```python
from build123d import *

# Parameters (mm, degrees)
SKETCH1_R           = 2
BOSS_EXTRUDE1_DEPTH = 8
SKETCH2_R           = 7.5
SKETCH2_R_2         = 4.5
BOSS_EXTRUDE2_DEPTH = 8
SKETCH3_R           = 2
BOSS_EXTRUDE3_DEPTH = 8
SKETCH8_W           = 30
SKETCH8_H           = 8
BOSS_EXTRUDE7_DEPTH = 15.35
BOSS_EXTRUDE8_DEPTH = 30
BOSS_EXTRUDE9_DEPTH = 8


with BuildPart() as part:
    # Sketch1 → Boss-Extrude1 (new body)
    with BuildSketch(Plane.XY):
        with BuildLine():
            Line((134.5, -11.9), (174.5, -11.9))
            ThreePointArc((174.5, -11.9), (182, -19.4), (174.5, -26.9))
            Line((174.5, -26.9), (134.5, -26.9))
            ThreePointArc((134.5, -26.9), (127, -19.4), (134.5, -11.9))
        make_face()
        with Locations((134.5, -19.4)):
            Circle(SKETCH1_R, mode=Mode.SUBTRACT)
        with Locations((174.5, -19.4)):
            Circle(SKETCH1_R, mode=Mode.SUBTRACT)
    extrude(amount=BOSS_EXTRUDE1_DEPTH)

    # Sketch8 → Boss-Extrude7 (add)
    with BuildSketch(Plane(origin=(0, -26.9, 0), x_dir=(-1, 0, 0), z_dir=(0, -1, 0))):
        with Locations((-154.2, -4)):
            Rectangle(SKETCH8_W, SKETCH8_H)
    extrude(amount=BOSS_EXTRUDE7_DEPTH)



with BuildPart() as body_2:
    # Sketch2 → Boss-Extrude2 (new body)
    with BuildSketch(Plane(origin=(0, -42.25, 0), x_dir=(1, 0, 0), z_dir=(0, 1, 0))):
        with Locations(Location((154.2, -16, 0), (0, 0, 270))):
            Circle(SKETCH2_R)
        with Locations(Location((154.2, -16, 0), (0, 0, 270))):
            Circle(SKETCH2_R_2, mode=Mode.SUBTRACT)
    extrude(amount=-BOSS_EXTRUDE2_DEPTH)

    # Sketch3 → Boss-Extrude3 (add)
    # profile 1 of 2: a face of its own
    with BuildSketch(Plane(origin=(0, -42.25, 0), x_dir=(1, 0, 0), z_dir=(0, 1, 0))):
        with BuildLine():
            Line((144.2, -11), (148.609830056, -11))
            ThreePointArc((148.609830056, -11), (146.7, -16), (148.609830056, -21))
            Line((148.609830056, -21), (144.2, -21))
            ThreePointArc((144.2, -21), (139.2, -16), (144.2, -11))
        make_face()
        with Locations(Location((144.2, -16, 0), (0, 0, 270))):
            Circle(SKETCH3_R, mode=Mode.SUBTRACT)
    # profile 2 of 2: a face of its own
    with BuildSketch(Plane(origin=(0, -42.25, 0), x_dir=(1, 0, 0), z_dir=(0, 1, 0))):
        with BuildLine():
            Line((164.2, -21), (159.790169944, -21))
            ThreePointArc((159.790169944, -21), (161.7, -16), (159.790169944, -11))
            Line((159.790169944, -11), (164.2, -11))
            ThreePointArc((164.2, -11), (169.2, -16), (164.2, -21))
        make_face()
        with Locations(Location((164.2, -16, 0), (0, 0, 90))):
            Circle(SKETCH3_R, mode=Mode.SUBTRACT)
    extrude(amount=-BOSS_EXTRUDE3_DEPTH)


with BuildPart() as part_1:
    add(part.part)

    add(body_2.part)  # Boss-Extrude8 merges body 2
    # Sketch9 → Boss-Extrude8 (add)
    with BuildSketch(Plane(origin=(169.2, 0, 0), x_dir=(0, 0, -1), z_dir=(1, 0, 0))):
        Polygon((-11, -50.25), (-8.5, -50.25), (0, -42.25), (-8, -42.25), (-11, -42.25), align=None)
    extrude(amount=-BOSS_EXTRUDE8_DEPTH)

    # Sketch10 → Boss-Extrude9 (add, through all)
    with BuildSketch(Plane(origin=(0, -42.25, 0), x_dir=(1, 0, 0), z_dir=(0, 1, 0))):
        with BuildLine():
            Line((139.2, -11), (139.2, -16))
            ThreePointArc((139.2, -16), (140.664466094, -12.464466094), (144.2, -11))
            Line((144.2, -11), (139.2, -11))
        make_face()
        with BuildLine():
            Line((169.2, -11), (164.2, -11))
            ThreePointArc((164.2, -11), (167.735533906, -12.464466094), (169.2, -16))
            Line((169.2, -16), (169.2, -11))
        make_face()
    extrude(amount=-BOSS_EXTRUDE9_DEPTH)


solid = part_1.part
```
Here's how the part is built. I have some questions about the finished solid (model axes, mm). A direction names the side the tool comes from. Coordinates: 2 decimals unless noted, no trailing zeros. Order: outer loops, then holes, each group sorted by start corner. A loop starts at its lowest first (then second) coordinate and runs counter-clockwise, first axis right, second up.
Item 1: If we section it at D-D, the plane z = 17: List the corners of the cut face in (x, y) for me.
Response values:
outline: (139.3, -50.25) - (142.47, -50.25) - (142.47, -42.25) - (139.3, -42.25) - close; (145.93, -50.25) - (149.81, -50.25) - (149.81, -42.25) - (145.93, -42.25) - close; (158.59, -50.25) - (162.47, -50.25) - (162.47, -42.25) - (158.59, -42.25) - close; (165.93, -50.25) - (169.1, -50.25) - (169.1, -42.25) - (165.93, -42.25) - close
Item 2: If we section it at C-C, the plane z = 19.5: List the corners of the cut face in (x, y) for me, then the cut area to 3 significant figures.
Response values:
outline: (140.63, -50.25) - (151.37, -50.25) - (151.37, -42.25) - (140.63, -42.25) - close; (157.03, -50.25) - (167.77, -50.25) - (167.77, -42.25) - (157.03, -42.25) - close
area: 172 mm2
Item 3: Thinking about a two-plate mould opening in Z: for faces 5 (the face through (151, -42.25, 12)), 6 (the face through (154.1, -46.2, 23.5)), 7 (the face through (157.24, -46.19, 12.68)), which applies, pulls with the +Z half, pulls with the -Z half, needs draft (parallel to the pull), parting line crosses it, or undercut?
Response values:
face 5: needs draft
face 6: pulls with the +Z half
face 7: undercut
Item 4: I'm going to push flat-ended pins straight in: pin 1 Ø3 at (x, z) = (170, 21) entering from -Y; pin 2 Ø15 at (x, y) = (142.5, -20) entering from +Z; pin 3 Ø5 at (x, y) = (163, -45.5) entering from +Z; pin 4 Ø4 at (x, z) = (136, 3.5) entering from -Y. Where does each tip first touch, or does it pass through?
Response values:
pin 1: passes through
pin 2: stops at z = 8
pin 3: stops at z = 21
pin 4: stops at y = -26.9
Item 5: Which directions (+Z, -Z, +X, -X, +Y, -Y) give clear straight access to the entire face, cutting with the end or side of a thin tool? Please do faces 1 (the face through (162, -46, 21)), 2 (the face through (169.2, -38, 6)), 3 (the face through (155, -23, 8)), 4 (the face through (146, -46, 21)).
Response values:
face 1: +Z, +X, +Y, -Y
face 2: +Z, -Z, +X, -Y
face 3: +Z, +X, -X, +Y
face 4: +Z, -X, +Y, -Y
Item 6: If we section it at B-B, the plane x = 152.5: List the corners of the cut face in (y, z) for me.
Response values:
outline: (-50.25, 8.5) - (-42.25, 0) - (-11.9, 0) - (-11.9, 8) - (-42.25, 8) - (-42.25, 11.83) - (-50.25, 11.83) - close; (-50.25, 20.17) - (-42.25, 20.17) - (-42.25, 23.3) - (-50.25, 23.3) - close
Item 7: If we section it at A-A, the plane y = -19.4: List the corners of the cut face in (x, z) for me, then the cut area to 3 significant figures.
Response values:
outline: (127, 0) - (132.5, 0) - (132.5, 8) - (127, 8) - close; (136.5, 0) - (172.5, 0) - (172.5, 8) - (136.5, 8) - close; (176.5, 0) - (182, 0) - (182, 8) - (176.5, 8) - close
area: 376 mm2
Item 8: I need wall thicknesses on probe 1 along X at (y, z) = (-48, 16); probe 2 along Y at (x, z) = (134.5, 4.75); probe 3 along Z at (x, y) = (148.5, -36). Which ranges of each line are inside material? Lowest first, please.
Response values:
probe 1: x = 139.2 to 142.2, 146.2 to 149.7, 158.7 to 162.2, 166.2 to 169.2
probe 2: y = -26.9 to -21.4, -17.4 to -11.9
probe 3: z = 0 to 8
